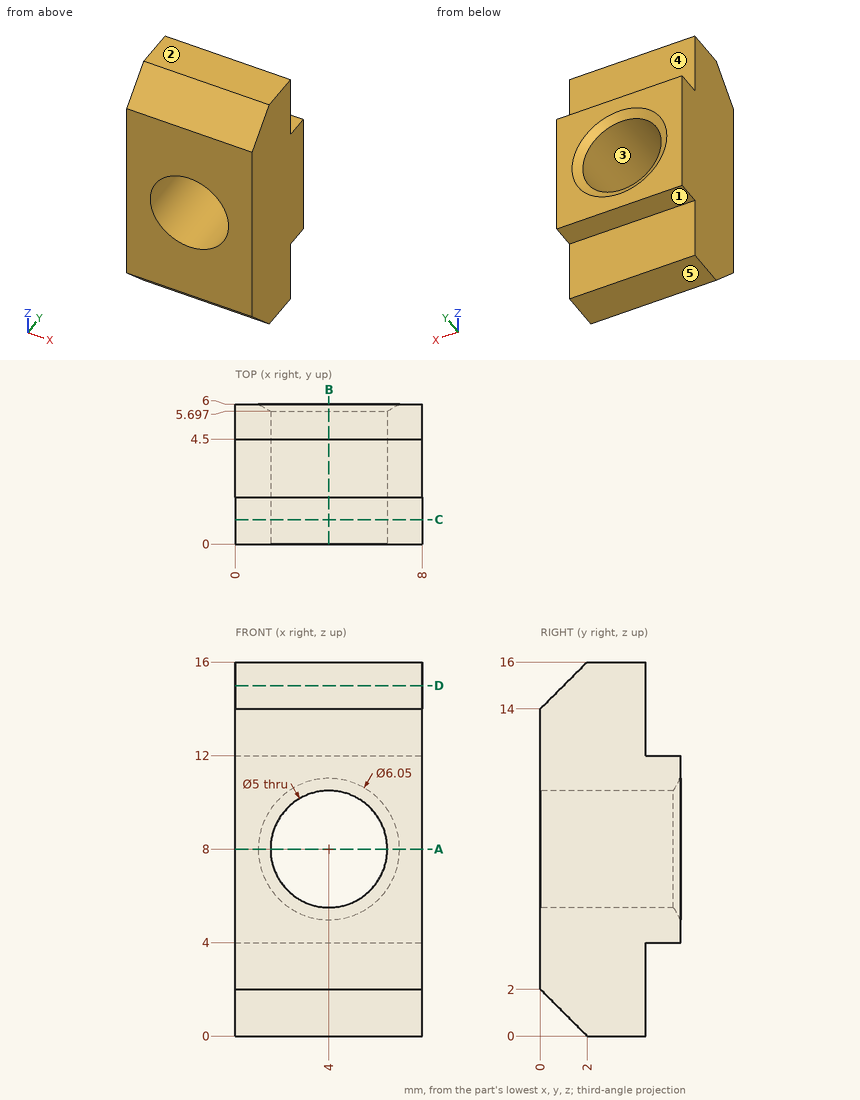
For this review, use the dimensioned drawing (mm, ordinates from the lowest corner) and the shaded views. A direction names the side the tool comes from. Round coordinates to 2 decimals unless told otherwise and drop trailing zeros. Order: outer loops, then holes, each group sorted by start corner. A loop starts at its lowest first (then second) coordinate and runs counter-clockwise, first axis right, second up. Notation, with made-up numbers: M 10,34.5 L 54,34.5 A12 ccw 54,56.5 Z; hole C -31.75,63.5 d4. An arc over 180 degrees is marked long. Use a Markdown table: item, result.
1) Consider section A-A (z = 8). Write out the cut boundary in (x, y) (3 decimals), then the cut area to 3 significant figures.
Report:
| item | result |
|---|---|
| outline | M 0,0 L 1.5,0 L 1.5,5.697 L 0.975,6 L 0,6 Z; M 6.5,0 L 8,0 L 8,6 L 7.025,6 L 6.5,5.697 Z |
| area | 17.8 mm^2 |
2) Draft analysis for pull direction Z (two halves, no side actions). For the marked faces 3, 4 and 5, state which applies: released by +Z, released by -Z, zero draft, split by the parting line, or undercut.
Report:
| item | result |
|---|---|
| face 3 | undercut |
| face 4 | zero draft |
| face 5 | released by -Z |
3) Consider section C-C (y = 1.05). Write out the cut boundary in (x, z).
Report:
| item | result |
|---|---|
| outline | M 0,0.95 L 8,0.95 L 8,15.05 L 0,15.05 Z; hole C 4,8 d5 |
4) Wall thickness on line 1 along X through (y, z) = (4.6, 9.5); line 2 along X through (y, z) = (2.45, 8); line 3 along Y through (x, z) = (2.75, 13.75): over which ranges is each line inside the solid? List them lowest first. Write a range as [from, to].
Report:
| item | result |
|---|---|
| line 1 | [0, 2], [6, 8] |
| line 2 | [0, 1.5], [6.5, 8] |
| line 3 | [0, 4.5] |
5) Consider section B-B (x = 4). Write out the cut boundary in (y, z) (3 decimals).
Report:
| item | result |
|---|---|
| outline | M 0,2 L 2,0 L 4.5,0 L 4.5,4 L 6,4 L 6,4.975 L 5.697,5.5 L 0,5.5 Z; M 0,10.5 L 5.697,10.5 L 6,11.025 L 6,12 L 4.5,12 L 4.5,16 L 2,16 L 0,14 Z |
6) Consider section D-D (z = 15). Write out the cut boundary in (x, y).
Report:
| item | result |
|---|---|
| outline | M 0,1 L 8,1 L 8,4.5 L 0,4.5 Z |
7) Insertion check: pin 1 (1.2 mm diameter, centred on x = 4.5, z = 2.5, fed in from +Y); pin 2 (1.5 mm diameter, centred on x = 5, z = 6, fed in from +Y). Each pin has a flat end and moves straight along its axis. Give the tip position at first contact, or say it passes through.
Report:
| item | result |
|---|---|
| pin 1 | y = 4.5 |
| pin 2 | y = 5.98 |
8) Tool access review of the marked faces 1 and 2: name each direction out of +Z, -Z, +X, -X, +Y, -Y from which nothing blocks a thin tool from reaching the whole face with its end or side.
Report:
| item | result |
|---|---|
| face 1 | -Z, +X, -X, +Y |
| face 2 | +Z, +X, -X, +Y, -Y |
